Check sheet for the modelled part. Datum: model origin and axes. Units: mm. Face numbers are marked on the shaded views. Give positions to 0.01 mm unless a question says otherwise; leave off trailing zeros. Write each loop counter-clockwise with the first axis right and the second up, starting at its lowest first coordinate (ties: lowest second). Pieces come first, ordered by that corner, then holes.
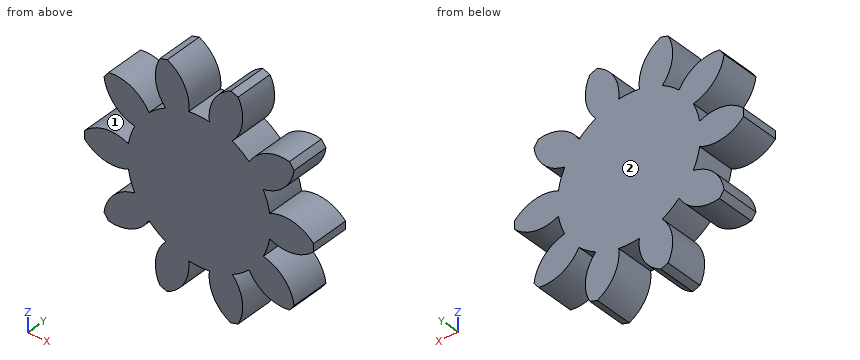
from build123d import *

# Parameters (mm, degrees)
SKETCH1_R           = 9
BOSS_EXTRUDE1_DEPTH = 3
CUT_EXTRUDE1_DEPTH  = 4
CIRPATTERN1_COUNT   = 10


with BuildPart() as part:
    # Sketch1 → Boss-Extrude1 (new body)
    with BuildSketch(Plane(origin=(0, 0, 0), x_dir=(1, 0, 0), z_dir=(0, 1, 0))):
        Circle(SKETCH1_R)
    extrude(amount=BOSS_EXTRUDE1_DEPTH)

    # Sketch2 → Cut-Extrude1 (cut, through all)
    with BuildSketch(Plane(origin=(0, 3, 0), x_dir=(1, 0, 0), z_dir=(0, 1, 0))):
        with BuildLine():
            ThreePointArc((-2.489254397, 8.648908171), (0, 9), (2.489254397, 8.648908171))
            ThreePointArc((2.489254397, 8.648908171), (1.152028564, 7.378729724), (0.810569881, 5.566291536))
            ThreePointArc((0.810569881, 5.566291536), (0, 5.625), (-0.810569881, 5.566291536))
            ThreePointArc((-0.810569881, 5.566291536), (-1.152028564, 7.378729724), (-2.489254397, 8.648908171))
        make_face()
    cut_extrude1 = extrude(amount=-CUT_EXTRUDE1_DEPTH, mode=Mode.SUBTRACT)

    # CirPattern1: Cut-Extrude1 ×10 about axis
    cirpattern1_axis = Axis((0, 0, 0), (0, 1, 0))
    for i in range(1, CIRPATTERN1_COUNT):
        add(cut_extrude1.rotate(cirpattern1_axis, i * 360 / CIRPATTERN1_COUNT), mode=Mode.SUBTRACT)


solid = part.part
1) Sectioned sample at D-D on z = -6. Record the boundary of the cut face in (x, y), then the cut area to 3 significant figures.
2) Sectioned sample at C-C on z = 5.25. Record the boundary of the cut face in (x, y), then the cut area to 3 significant figures.
3) Draft check along Z on the marked faces 1 and 2. Enter one of: +Z half, -Z half, draft (parallel to the pull), parting line (faces both ways), or undercut.
4) Scan lines: L1, parallel to Z at x = -2.75, y = 0.85; L2, parallel to Z at x = 7, y = 1.05; L3, parallel to X at y = 1.3, z = 5.25. Record each from-to range of solid material in increasing order.
5) Sectioned sample at B-B on x = 6.75. Record the boundary of the cut face in (y, z).
6) Gauge pin test, flat ends, axial feed: pin 1 (1 mm diameter, centred on y = 2, z = 2, fed in from -X); pin 2 (2 mm diameter, centred on x = -5, z = 6.5, fed in from +Y). Record the tip position at first contact, or that the pin passes through.
7) Sectioned sample at A-A on z = 7.5. Record the boundary of the cut face in (x, y).
Answers below:
1. outline: (-3.25, 0) - (-0.79, 0) - (-0.79, 3) - (-3.25, 3) - close; (0.79, 0) - (3.25, 0) - (3.25, 3) - (0.79, 3) - close
1. area: 14.8 mm2
2. outline: (-7.31, 0) - (-5.18, 0) - (-5.18, 3) - (-7.31, 3) - close; (-2.84, 0) - (2.84, 0) - (2.84, 3) - (-2.84, 3) - close; (5.18, 0) - (7.31, 0) - (7.31, 3) - (5.18, 3) - close
2. area: 29.8 mm2
3. face 1: undercut
3. face 2: draft
4. L1: z = -8.57 to -5.13, -4.91 to 4.91, 5.13 to 8.57
4. L2: z = -5.55 to -3.81, -1.23 to 1.23, 3.81 to 5.55
4. L3: x = -7.31 to -5.18, -2.84 to 2.84, 5.18 to 7.31
5. outline: (0, -5.58) - (3, -5.58) - (3, -3.47) - (0, -3.47) - close; (0, -1.23) - (3, -1.23) - (3, 1.23) - (0, 1.23) - close; (0, 3.47) - (3, 3.47) - (3, 5.58) - (0, 5.58) - close
6. pin 1: stops at x = -5.42
6. pin 2: passes through
7. outline: (-3.39, 0) - (-1.22, 0) - (-1.22, 3) - (-3.39, 3) - close; (1.22, 0) - (3.39, 0) - (3.39, 3) - (1.22, 3) - close
